```python
from build123d import *

# Parameters (mm, degrees)
F0_W     = 10
F0_H     = 20
F1_DEPTH = 25
F3_DEPTH = 10.001
F4_R     = 3.75
F5_DEPTH = 12.5
F7_D     = 4.2
F7_DEPTH = 14.4
F7_TIP   = 1.2618073


with BuildPart() as f1:
    # F0 (on Top) → F1 (new body)
    with BuildSketch(Plane.XY):
        Polygon((0, -22.2465131165), (5, -3.5862590786), (-5, -3.5862590786), align=None)
        with Locations((0, 6.4137409214)):
            Rectangle(F0_W, F0_H)
        with BuildLine():
            Line((-5, 16.4137409214), (5, 16.4137409214))
            ThreePointArc((5, 16.4137409214), (0, 21.4137409214), (-5, 16.4137409214))
        make_face()
    extrude(amount=F1_DEPTH)

    # F2 (on face) → F3 (cut, through all)
    with BuildSketch(Plane.YZ.offset(5)):
        Polygon((11.4137409214, 12.5), (6.4137409214, 18.75), (1.4137409214, 12.5), (6.4137409214, 6.25), align=None)
    extrude(amount=-F3_DEPTH, mode=Mode.SUBTRACT)

    # F4 (on Right) → F5 (cut, symmetric)
    with BuildSketch(Plane.YZ):
        with Locations((-12.9163860975, 12.5)):
            Circle(F4_R)
    extrude(amount=F5_DEPTH, both=True, mode=Mode.SUBTRACT)

    # F7
    with Locations(Plane.XY.offset(25)):
        with Locations((0, 16.4137409214)):
            Hole(F7_D / 2, depth=F7_DEPTH)
            with Locations((0, 0, -(F7_DEPTH + F7_TIP / 2))):  # 118° drill point
                Cone(0, F7_D / 2, F7_TIP, mode=Mode.SUBTRACT)


solid = f1.part
```
For this review, take the finished solid that the model builds, in its own axes (mm). A direction names the side the tool comes from. Give positions to 0.01 mm unless a question says otherwise; leave off trailing zeros. Order: outer loops, then holes, each group sorted by start corner. A loop starts at its lowest first (then second) coordinate and runs counter-clockwise, first axis right, second up.
1) Take a section at C-C (z = 22.75). Give the boundary of the cut face in (x, y).
2) Take a section at B-B (y = -16). Give the boundary of the cut face in (x, z).
3) For faces 5 (the face through (-1.129, 18.184, 17.699)), 6 (the face through (5, 2, 10)), 7 (the face through (0.07, 8.88, 9.33)), list the 3-axis set-ups (+Z, -Z, +X, -X, +Y, -Y) from which the entire face can be reached by the end or side of a thin tool; tool diameter is ignored.
4) Take a section at A-A (z = 13.25). Give the boundary of the cut face in (x, y), then the cut area to 3 significant figures.
5) Wall thickness on line 1 (X direction, y = 16.5, z = 22); line 2 (Y direction, x = -3, z = 15.5); line 3 (Z direction, x = 0.5, y = -14.5): over which ranges is each line inside the solid? List them lowest first.
6) Insertion check: pin 1 (1.5 mm diameter, centred on x = 3, z = 12, fed in from +Y); pin 2 (1 mm diameter, centred on y = -15, z = 18, fed in from -X); pin 3 (5 mm diameter, centred on x = 4, z = 5.5, fed in from +Y). Each pin has a flat end and moves straight along its axis. Give the tip position at first contact, or say it passes through.
7) Take a section at D-D (z = 4.75). Give the boundary of the cut face in (x, y), then the cut area to 3 significant figures.
8) The part is to be moulded in two halves that separate along Y. For faces 1 (the face through (0.05, -9.34, 13.63)), 2 (the face through (3.576, -8.9, 12.325)), 3 (the face through (0, 5, 25)), 4 (the face through (0.07, 3.88, 9.42)), say which applies: released by +Y, released by -Y, zero draft, split by the parting line, or undercut.
Derived:
1. outline: (-5, -3.59) - (0, -22.25) - (5, -3.59) - (5, 16.41) arc R5 ccw to (-5, 16.41) - close; hole circle Ø4.2 at (0, 16.41)
2. outline: (-1.67, 0) - (1.67, 0) - (1.67, 10.37) - (-1.67, 10.37) - close; (-1.67, 14.63) - (1.67, 14.63) - (1.67, 25) - (-1.67, 25) - close
3. face 5: +Z
3. face 6: +Z, -Z, +X, +Y, -Y
3. face 7: +X, -X
4. outline: (-5, -3.59) - (-3.48, -9.24) - (3.48, -9.24) - (5, -3.59) - (5, 2.01) - (-5, 2.01) - close; (-5, 10.81) - (5, 10.81) - (5, 16.41) arc R5 ccw to (-5, 16.41) - close; (-1.52, -16.59) - (0, -22.25) - (1.52, -16.59) - close; hole circle Ø4.2 at (0, 16.41)
4. area: 194 mm2
5. line 1: x = -5 to -2.1, 2.1 to 5
5. line 2: y = -10.67 to 3.81, 9.01 to 20.41
5. line 3: z = 0 to 9.1, 15.9 to 25
6. pin 1: stops at y = 20.88
6. pin 2: stops at x = -2.08
6. pin 3: stops at y = 21.18
7. outline: (-5, -3.59) - (0, -22.25) - (5, -3.59) - (5, 16.41) arc R5 ccw to (-5, 16.41) - close
7. area: 333 mm2
8. face 1: undercut
8. face 2: released by -Y
8. face 3: zero draft
8. face 4: undercut
